Check sheet for the modelled part. Datum: model origin and axes. Units: mm. Face numbers are marked on the shaded views. A direction names the side the tool comes from. Coordinates: 2 decimals unless noted, no trailing zeros. Loops run counter-clockwise (first coordinate to the right, second up) from the corner with the lowest first, then second, coordinate; pieces in that order, holes last. Notation, with made-up numbers: M -20.75,21.25 L -10.75,21.25 A29 cw -10.75,44.25 Z; hole C 67.25,-40 d3. An arc over 180 degrees is marked long. Use CSV: the item, a comma, the result in double quotes. Start each with the question number.
(1) Draft check along X on the marked faces 1, 2, 3 and 4. Enter one of: pulls with the +X half, pulls with the -X half, needs draft (parallel to the pull), parting line crosses it, or undercut.
(2) Section check C-C on y = 7.25. Record the cut outline in (x, z) (3 decimals).
(3) Section check A-A on z = 0. Record the cut outline in (x, y) (3 decimals).
(4) Set-up check for the marked faces 5, 6, 7 and 8: record each of +Z, -Z, +X, -X, +Y, -Y from which the full face is reachable in a straight line by a thin tool's end or side.
(5) Scan lines: line 1 (X direction, y = 13.45, z = 0) (3 decimals); line 2 (X direction, y = 9, z = -1.75) (3 decimals); line 3 (Z direction, x = 8.5, y = 6.75). Record each from-to range of solid material in increasing order.
(6) Go/stop test with flat-tipped pins: pin 1 Ø2 at (y, z) = (8.5, 3) entering from -X (3 decimals); pin 2 Ø3 at (y, z) = (9.5, -3) entering from +X; pin 3 Ø3.5 at (y, z) = (9.5, 0.5) entering from -X. Record where each tip stops, or that it passes through.
(7) Section check B-B on y = 13.5. Record the cut outline in (x, z) (3 decimals), and give its area (3 significant figures).
(8) Section check D-D on x = 10. Record the cut outline in (y, z), and give its area (4 significant figures).
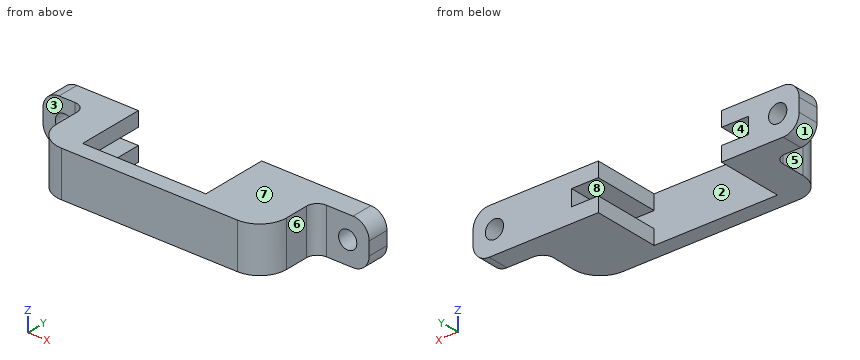
from build123d import *

# Parameters (mm, degrees)
SKETCH1_W           = 60.85
SKETCH1_H           = 8.5
BOSS_EXTRUDE1_DEPTH = 15.5
SKETCH4_R           = 1.7
CUT_EXTRUDE3_DEPTH  = 35.409201168
SKETCH2_W           = 5
SKETCH2_H           = 3
CUT_EXTRUDE1_DEPTH  = 12.5
SKETCH3_W           = 8
SKETCH3_H           = 8.5
SKETCH3_W_2         = 10
CUT_EXTRUDE2_DEPTH  = 11.5
FILLET1_R           = 2
FILLET2_R           = 3
FILLET3_R           = 5


with BuildPart() as part:
    # Sketch1 → Boss-Extrude1 (new body)
    with BuildSketch(Plane(origin=(0, 0, 0), x_dir=(1, 0, 0), z_dir=(0, 1, 0))):
        Rectangle(SKETCH1_W, SKETCH1_H)
    extrude(amount=BOSS_EXTRUDE1_DEPTH)

    # Sketch4 → Cut-Extrude3 (cut, through all)
    with BuildSketch(Plane(origin=(0, 15.5, 0), x_dir=(1, 0, 0), z_dir=(0, 1, 0))):
        with Locations(Location((-26.425, 0, 0), (0, 0, 270))):
            Circle(SKETCH4_R)
        with Locations(Location((26.425, 0, 0), (0, 0, 90))):
            Circle(SKETCH4_R)
    extrude(amount=-CUT_EXTRUDE3_DEPTH, mode=Mode.SUBTRACT)

    # Sketch2 → Cut-Extrude1 (cut)
    with BuildSketch(Plane(origin=(0, 15.5, 0), x_dir=(1, 0, 0), z_dir=(0, 1, 0))):
        Polygon((-15.96, -1.5), (-15.96, -4.25), (7.04, -4.25), (7.04, -1.5), (7.04, 1.5), (7.04, 4.25), (-15.96, 4.25), (-15.96, 1.5), align=None)
        with Locations((-18.46, 0)):
            Rectangle(SKETCH2_W, SKETCH2_H)
        with Locations((9.54, 0)):
            Rectangle(SKETCH2_W, SKETCH2_H)
    extrude(amount=-CUT_EXTRUDE1_DEPTH, mode=Mode.SUBTRACT)

    # Sketch3 → Cut-Extrude2 (cut)
    with BuildSketch(Plane.XZ):
        with Locations((-26.425, 0)):
            Rectangle(SKETCH3_W, SKETCH3_H)
        with Locations((25.425, 0)):
            Rectangle(SKETCH3_W_2, SKETCH3_H)
    extrude(amount=-CUT_EXTRUDE2_DEPTH, mode=Mode.SUBTRACT)

    # Fillet1
    fillet1_edges = [part.edges().sort_by_distance(p)[0] for p in [
        (-22.425, 11.5, 0),
        (20.425, 11.5, 0),
    ]]
    fillet(fillet1_edges, radius=FILLET1_R)

    # Fillet2
    fillet2_edges = [part.edges().sort_by_distance(p)[0] for p in [
        (30.425, 13.5, 4.25),
        (-30.425, 13.5, 4.25),
        (-30.425, 13.5, -4.25),
        (30.425, 13.5, -4.25),
    ]]
    fillet(fillet2_edges, radius=FILLET2_R)

    # Fillet3
    fillet3_edges = [part.edges().sort_by_distance(p)[0] for p in [
        (-22.425, 0, 0),
        (20.425, 0, 0),
    ]]
    fillet(fillet3_edges, radius=FILLET3_R)


solid = part.part
Outcome:
1,face 1,"pulls with the -X half"
1,face 2,"undercut"
1,face 3,"needs draft"
1,face 4,"undercut"
2,outline,"M -22.425,-4.25 L -15.96,-4.25 L -15.96,-1.5 L -20.96,-1.5 L -20.96,1.5 L -15.96,1.5 L -15.96,4.25 L -22.425,4.25 Z; M 7.04,-4.25 L 20.425,-4.25 L 20.425,4.25 L 7.04,4.25 L 7.04,1.5 L 12.04,1.5 L 12.04,-1.5 L 7.04,-1.5 Z"
3,outline,"M -30.425,11.5 L -28.125,11.5 L -28.125,15.5 L -30.425,15.5 Z; M -24.725,11.5 L -24.425,11.5 A2 cw -22.425,9.5 L -22.425,5 A5 ccw -17.425,0 L 15.425,0 A5 ccw 20.425,5 L 20.425,9.5 A2 cw 22.425,11.5 L 24.725,11.5 L 24.725,15.5 L 12.04,15.5 L 12.04,3 L -20.96,3 L -20.96,15.5 L -24.725,15.5 Z; M 28.125,11.5 L 30.425,11.5 L 30.425,15.5 L 28.125,15.5 Z"
4,face 5,"+Z, -Z, -X, -Y"
4,face 6,"+Z, -Z, +X, -Y"
4,face 7,"+Z, +X, -X, +Y, -Y"
4,face 8,"+Y"
5,line 1,"x = -30.425 to -28.125, -24.725 to -20.96, 12.04 to 24.725, 28.125 to 30.425"
5,line 2,"x = -22.425 to -15.96, 7.04 to 20.425"
5,line 3,"z = -4.25 to -1.5, 1.5 to 4.25"
6,pin 1,"stops at x = -22.425"
6,pin 2,"stops at x = 21.1"
6,pin 3,"stops at x = -23.46"
7,outline,"M -30.425,-1.25 A3 ccw -27.425,-4.25 L -15.96,-4.25 L -15.96,-1.5 L -20.96,-1.5 L -20.96,1.5 L -15.96,1.5 L -15.96,4.25 L -27.425,4.25 A3 ccw -30.425,1.25 Z; M 7.04,-4.25 L 27.425,-4.25 A3 ccw 30.425,-1.25 L 30.425,1.25 A3 ccw 27.425,4.25 L 7.04,4.25 L 7.04,1.5 L 12.04,1.5 L 12.04,-1.5 L 7.04,-1.5 Z; hole C -26.425,0 d3.4; hole C 26.425,0 d3.4"
7,area,"266 mm²"
8,outline,"M 0,-4.25 L 15.5,-4.25 L 15.5,-1.5 L 3,-1.5 L 3,1.5 L 15.5,1.5 L 15.5,4.25 L 0,4.25 Z"
8,area,"94.25 mm²"
